Print and shaded views of the part. All mm, measured from the part's lowest x, y and z. Round coordinates to 2 decimals unless told otherwise and drop trailing zeros. Loops run counter-clockwise (first coordinate to the right, second up) from the corner with the lowest first, then second, coordinate; pieces in that order, holes last. Notation, with made-up numbers: (37, -37.5) - (80, -37.5) arc R33 cw to (80, -7.5) - close; hole circle Ø5 at (10, 76). An arc over 180 degrees is marked (long way). Put each result on its own line as item: value. Start each with the question number.
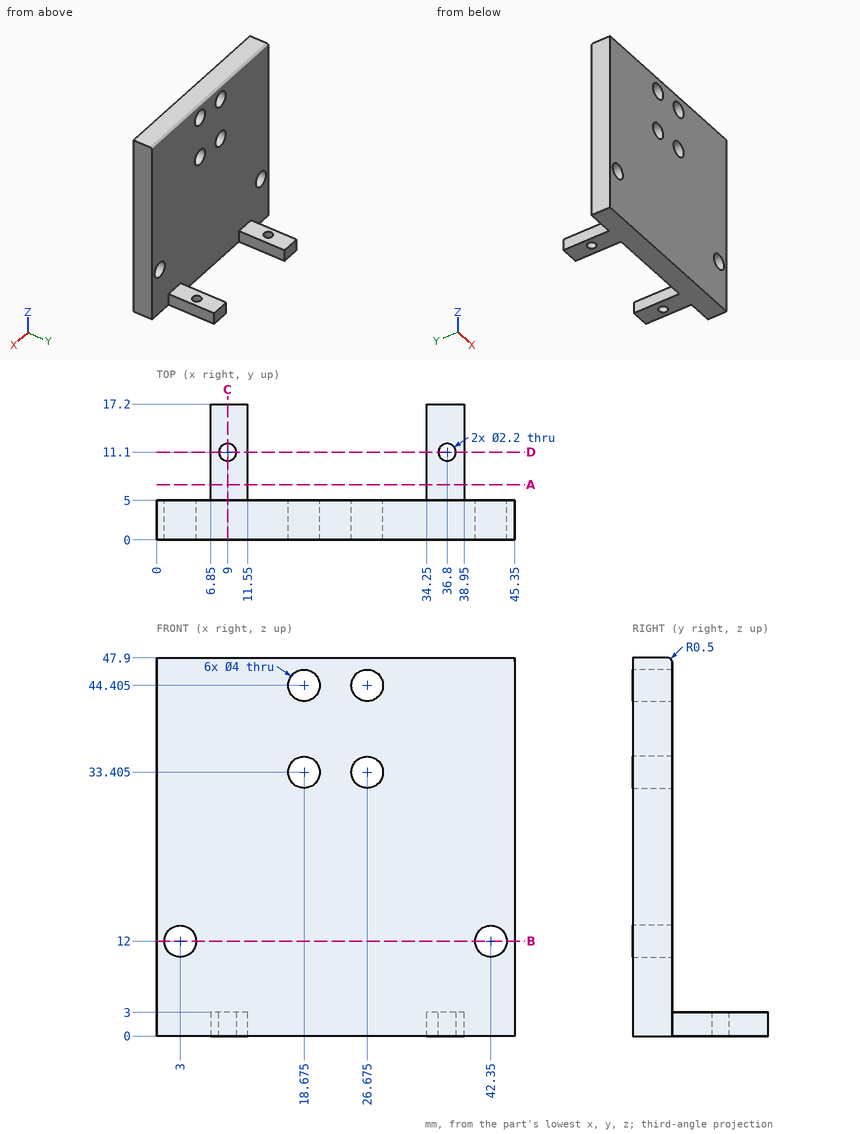
Item 1: Slice it at D-D (y = 11.1). Give the cut face in (x, z), plus the area to 3 significant figures.
Item 2: Slice it at C-C (x = 9). Give the cut face in (y, z).
Item 3: Slice it at A-A (y = 7). Give the cut face in (x, z).
Item 4: Drill centre lines: probe 1 along Y at (x, z) = (36.8, 0.8); probe 2 along Z at (x, y) = (27.5, 4.5); probe 3 along Y at (x, z) = (18, 9). Where is each one in solid material? Low to high. Write a range as [from, to].
Item 5: Slice it at B-B (z = 12). Give the cut face in (x, y), plus the area to 3 significant figures.
Item 6: Drop flat-ended pins along their axis: pin 1 Ø10 at (x, z) = (31, 19.5) entering from -Y; pin 2 Ø3 at (x, z) = (26.68, 44.4) entering from +Y; pin 3 Ø4 at (x, z) = (36, 35.5) entering from +Y; pin 4 Ø1.5 at (y, z) = (10.5, 1.5) entering from +X. Give the stop position or say it passes through.
Computed values:
1. outline: (6.85, 0) - (7.9, 0) - (7.9, 3) - (6.85, 3) - close; (10.1, 0) - (11.55, 0) - (11.55, 3) - (10.1, 3) - close; (34.25, 0) - (35.7, 0) - (35.7, 3) - (34.25, 3) - close; (37.9, 0) - (38.95, 0) - (38.95, 3) - (37.9, 3) - close
1. area: 15.0 mm^2
2. outline: (0, 0) - (10, 0) - (10, 3) - (5, 3) - (5, 47.4) arc R0.5 ccw to (4.5, 47.9) - (0, 47.9) - close; (12.2, 0) - (17.2, 0) - (17.2, 3) - (12.2, 3) - close
3. outline: (6.85, 0) - (11.55, 0) - (11.55, 3) - (6.85, 3) - close; (34.25, 0) - (38.95, 0) - (38.95, 3) - (34.25, 3) - close
4. probe 1: y = [0, 10], [12.2, 17.2]
4. probe 2: z = [0, 31.58], [35.23, 42.58], [46.23, 47.9]
4. probe 3: y = [0, 5]
5. outline: (0, 0) - (1, 0) - (1, 5) - (0, 5) - close; (5, 0) - (40.35, 0) - (40.35, 5) - (5, 5) - close; (44.35, 0) - (45.35, 0) - (45.35, 5) - (44.35, 5) - close
5. area: 187 mm^2
6. pin 1: stops at y = 0
6. pin 2: passes through
6. pin 3: stops at y = 5
6. pin 4: stops at x = 38.95
